from build123d import *

# Parameters (mm, degrees)
SKETCH1_W           = 37
SKETCH1_H           = 3.6
BOSS_EXTRUDE1_DEPTH = 3.6
SKETCH2_R           = 0.8
CUT_EXTRUDE1_DEPTH  = 3.6
SKETCH3_R           = 0.8
CUT_EXTRUDE2_DEPTH  = 3.6


with BuildPart() as part:
    # Sketch1 → Boss-Extrude1 (new body)
    with BuildSketch(Plane.XY):
        with Locations((-23.279872622, 10.227539088)):
            Rectangle(SKETCH1_W, SKETCH1_H)
    extrude(amount=BOSS_EXTRUDE1_DEPTH)

    # Sketch2 → Cut-Extrude1 (cut)
    with BuildSketch(Plane.XY.offset(3.6)):
        with Locations((-6.379872622, 10.227539088)):
            Circle(SKETCH2_R)
    extrude(amount=-CUT_EXTRUDE1_DEPTH, mode=Mode.SUBTRACT)

    # Sketch3 → Cut-Extrude2 (cut)
    with BuildSketch(Plane.XZ.offset(-8.427539088)):
        with Locations(Location((-40.179872622, 2, 0), (0, 0, 270))):
            Circle(SKETCH3_R)
    extrude(amount=-CUT_EXTRUDE2_DEPTH, mode=Mode.SUBTRACT)


solid = part.part
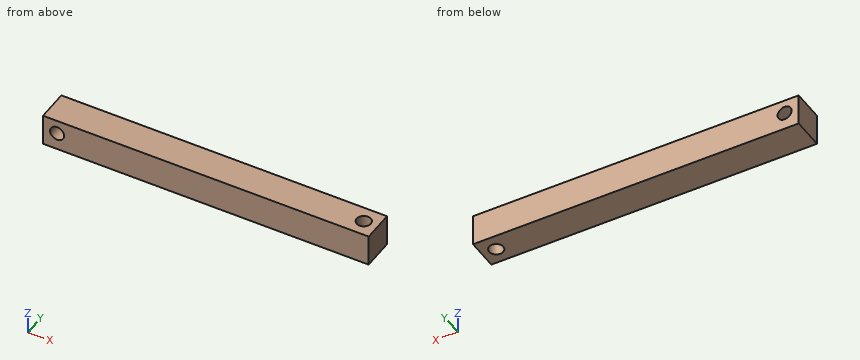
CAD build for the part. Positions are in the model's coordinates, mm. Give positions to 0.01 mm unless a question says otherwise; leave off trailing zeros. Write each loop counter-clockwise with the first axis right and the second up, starting at its lowest first coordinate (ties: lowest second). Pieces come first, ordered by that corner, then holes. Notation, with made-up numbers: (30, 37.25) - (53, 37.25) arc R19 ccw to (53, 73.25) - close; hole circle Ø10 at (20.25, 28.25). An arc over 180 degrees is marked (long way). Put each result on its own line as item: value.
(1) Saw through at B-B (y = 9.8). List the corners of the cut face in (x, z), then the cut area to 3 significant figures.
Working result:
outline: (-41.78, 0) - (-7.06, 0) - (-7.06, 3.6) - (-41.78, 3.6) - close; (-5.7, 0) - (-4.78, 0) - (-4.78, 3.6) - (-5.7, 3.6) - close; hole circle Ø1.6 at (-40.18, 2)
area: 126 mm^2
(2) Saw through at A-A (z = 2). List the corners of the cut face in (x, y), then the cut area to 3 significant figures.
Working result:
outline: (-41.78, 8.43) - (-40.98, 8.43) - (-40.98, 12.03) - (-41.78, 12.03) - close; (-39.38, 8.43) - (-4.78, 8.43) - (-4.78, 12.03) - (-39.38, 12.03) - close; hole circle Ø1.6 at (-6.38, 10.23)
area: 125 mm^2
(3) Wall check: L1, parallel to X at y = 10.4, z = 1.65; L2, parallel to X at y = 10.25, z = 0.3; L3, parallel to X at y = 10.8, z = 2. Give the ranges that are in metal, low to high.
Working result:
L1: -41.78 to -40.9, -39.46 to -7.16, -5.6 to -4.78
L2: -41.78 to -7.18, -5.58 to -4.78
L3: -41.78 to -40.98, -39.38 to -6.94, -5.82 to -4.78
